from build123d import *

# Parameters (mm, degrees)
BOSS_EXTRUDE1_DEPTH = 25.4
SKETCH2_R           = 4.389630664
BOSS_EXTRUDE4_DEPTH = 25.4
CUT_EXTRUDE1_START  = -25.4
SKETCH4_R           = 4.389630664
CUT_EXTRUDE1_DEPTH  = 25.4
SKETCH6_R           = 4.445
CUT_EXTRUDE2_DEPTH  = 25.4
SKETCH7_W           = 50.8
SKETCH7_H           = 774.7
BOSS_EXTRUDE5_DEPTH = 25.4
SKETCH8_R           = 4.445
CUT_EXTRUDE3_DEPTH  = 50.8


with BuildPart() as part:
    # Sketch1 → Boss-Extrude1 (new body)
    with BuildSketch(Plane(origin=(0, 0, 0), x_dir=(0, 0, -1), z_dir=(1, 0, 0))):
        Polygon((-50.8, 774.7), (-454.899551596, 0), (-404.099551596, 0), (0, 774.7), align=None)
    extrude(amount=BOSS_EXTRUDE1_DEPTH)

    # Sketch2 → Boss-Extrude4 (add)
    with BuildSketch(Plane(origin=(0, 0, 0), x_dir=(0, 0, -1), z_dir=(1, 0, 0))):
        Polygon((0, 0), (-333.48251995, 174.895038051), (-363.670680481, 174.895038051), (-368.098145545, 166.407136563), (-50.8, 0), align=None)
        with Locations((-333.48251995, 161.772531454)):
            Circle(SKETCH2_R, mode=Mode.SUBTRACT)
    extrude(amount=-BOSS_EXTRUDE4_DEPTH)

    # Sketch4 → Cut-Extrude1 (cut)
    with BuildSketch(Plane.ZY.offset(CUT_EXTRUDE1_START)):
        with Locations(Location((333.48251995, 161.772531454, 0), (0, 0, 180))):
            Circle(SKETCH4_R)
    extrude(amount=CUT_EXTRUDE1_DEPTH, mode=Mode.SUBTRACT)

    # Sketch6 → Cut-Extrude2 (cut)
    with BuildSketch(Plane.ZY):
        with Locations((417.660059318, 8.400584223)):
            Circle(SKETCH6_R)
    extrude(amount=-CUT_EXTRUDE2_DEPTH, mode=Mode.SUBTRACT)

    # Sketch7 → Boss-Extrude5 (add)
    with BuildSketch(Plane.ZY):
        with Locations((25.4, 387.35)):
            Rectangle(SKETCH7_W, SKETCH7_H)
    extrude(amount=BOSS_EXTRUDE5_DEPTH)

    # Sketch8 → Cut-Extrude3 (cut)
    with BuildSketch(Plane(origin=(25.4, 0, 0), x_dir=(0, 0, -1), z_dir=(1, 0, 0))):
        with Locations((-32.253882692, 739.883035965)):
            Circle(SKETCH8_R)
    extrude(amount=-CUT_EXTRUDE3_DEPTH, mode=Mode.SUBTRACT)


solid = part.part
Geometry check sheet. Reference: the model listing, model coordinates, mm. A direction names the side the tool comes from. Round coordinates to 2 decimals unless told otherwise and drop trailing zeros. Order: outer loops, then holes, each group sorted by start corner. A loop starts at its lowest first (then second) coordinate and runs counter-clockwise, first axis right, second up. Notation, with made-up numbers: M -25,-15 L 12,-15 A20 ccw 12,-6 Z; hole C 36,38 d3. An arc over 180 degrees is marked long. Write each question's results on one line, items separated by ' | '. Start each with the question number.
1. Go/stop test with flat-tipped pins: P1, Ø6, axis at x = 16, y = 154, coming from the -Z side; P2, Ø11.5, axis at y = 8.4, z = 417.66, coming from the +X side; P3, Ø5, axis at x = 10, y = 271.5, coming from the -Z side; P4, Ø2, axis at x = -14.5, y = 591.5, coming from the +Z side. Record where each tip stops, or that it passes through.
2. Material ranges on L1, parallel to Z at x = -21.5, y = 698.5; L2, parallel to X at y = 264.5, z = 280.5; L3, parallel to Z at x = -15.5, y = 153.5, recorded low to high. Write a range as from..to.
3. Cross-section at C-C on z = 108. Record the boundary of the cut face in (x, y).
4. Cross-section at D-D on x = -12. Record the boundary of the cut face in (y, z) (3 decimals).
5. Set-up check for faces 1 (the face through (-13, 174.895, 348)), 2 (the face through (0, 77, 387)), 3 (the face through (13, 0, 430)), 4 (the face through (0, 303, 42)): record each of +Z, -Z, +X, -X, +Y, -Y from which the full face is reachable in a straight line by a thin tool's end or side.
6. Cross-section at B-B on y = 262. Record the boundary of the cut face in (x, z).
7. Draft check along Z on faces 5 (the face through (-25.4, 332, 47)), 6 (the face through (-13, 395, 50.8)), 7 (the face through (-12.52, 84.37, 211.67)). Enter one of: pulls with the +Z half, pulls with the -Z half, needs draft (parallel to the pull), parting line crosses it, or undercut.
8. Cross-section at A-A on y = 98.5. Record the boundary of the cut face in (x, z).
Resolved:
1) P1: z = 322.21 | P2: x = 25.4 | P3: z = 261.18 | P4: z = 50.8
2) L1: 0..50.8 | L2: 0..25.4 | L3: 0..50.8, 292.69..343.49
3) outline: M -25.4,30 L 0,30 L 0,56.64 L -25.4,56.64 Z; M 0,567.65 L 25.4,567.65 L 25.4,665.04 L 0,665.04 Z
4) outline: M 0,0 L 774.7,0 L 774.7,50.8 L 26.642,50.8 L 174.895,333.483 L 174.895,363.671 L 166.407,368.098 L 0,50.8 Z; hole C 161.773,333.483 d8.779; hole C 739.883,32.254 d8.89
5) face 1: +Z, -X, +Y | face 2: +Z, -X, -Y | face 3: +Z, -Z, +X, -X, -Y | face 4: -Z, +X, -Y
6) outline: M -25.4,0 L 0,0 L 0,50.8 L -25.4,50.8 Z; M 0,267.43 L 25.4,267.43 L 25.4,318.23 L 0,318.23 Z
7) face 5: needs draft | face 6: undercut | face 7: pulls with the +Z half
8) outline: M -25.4,0 L 0,0 L 0,50.8 L -25.4,50.8 Z; M -25.4,187.82 L 0,187.82 L 0,238.62 L -25.4,238.62 Z; M 0,352.72 L 25.4,352.72 L 25.4,403.52 L 0,403.52 Z
